```python
from build123d import *

# Parameters (mm, degrees)
SKETCH1_R                      = 88.9
BOSS_EXTRUDE1_DEPTH            = 3.175
SKETCH2_R                      = 12.065
BOSS_EXTRUDE2_DEPTH            = 3.175
SKETCH5_R                      = 10.4
CUT_EXTRUDE1_DEPTH             = 5.525
SKETCH6_R                      = 5
CUT_EXTRUDE2_DEPTH             = 4
CBORE_FOR_M2_SHCS1_D           = 2.2
CBORE_FOR_M2_SHCS1_DEPTH       = 6
CBORE_FOR_M2_SHCS1_CBORE_D     = 4.4
CBORE_FOR_M2_SHCS1_CBORE_DEPTH = 2
CBORE_FOR_M2_SHCS1_TIP         = 0.660946681
M4_CLEARANCE_HOLE1_D           = 4.5
CHAMFER1_SIZE                  = 5.08


with BuildPart() as part:
    # Sketch1 → Boss-Extrude1 (new, symmetric)
    with BuildSketch(Plane(origin=(0, 0, 0), x_dir=(1, 0, 0), z_dir=(0, 1, 0))):
        with Locations(Location((0, 0, 0), (0, 0, 270))):
            Circle(SKETCH1_R)
    extrude(amount=BOSS_EXTRUDE1_DEPTH, both=True)

    # Sketch2 → Boss-Extrude2 (add)
    with BuildSketch(Plane.XZ.offset(3.175)):
        with Locations(Location((0, 0, 0), (0, 0, 90))):
            Circle(SKETCH2_R)
    extrude(amount=BOSS_EXTRUDE2_DEPTH)

    # Sketch5 → Cut-Extrude1 (cut)
    with BuildSketch(Plane(origin=(0, 3.175, 0), x_dir=(1, 0, 0), z_dir=(0, 1, 0))):
        with Locations(Location((0, 0, 0), (0, 0, 270))):
            Circle(SKETCH5_R)
    extrude(amount=-CUT_EXTRUDE1_DEPTH, mode=Mode.SUBTRACT)

    # Sketch6 → Cut-Extrude2 (cut)
    with BuildSketch(Plane(origin=(0, -2.35, 0), x_dir=(1, 0, 0), z_dir=(0, 1, 0))):
        with Locations(Location((0, 0, 0), (0, 0, 270))):
            Circle(SKETCH6_R)
    extrude(amount=-CUT_EXTRUDE2_DEPTH, mode=Mode.SUBTRACT)

    # CBORE for M2 SHCS1
    with Locations(Plane(origin=(0, -2.35, 0), x_dir=(1, 0, 0), z_dir=(0, 1, 0))):
        with Locations((-5.65685425, 5.65685425), (0, 8), (5.65685425, 5.65685425), (8, 0), (5.65685425, -5.65685425), (0, -8), (-5.65685425, -5.65685425), (-8, 0)):
            CounterBoreHole(CBORE_FOR_M2_SHCS1_D / 2, CBORE_FOR_M2_SHCS1_CBORE_D / 2, CBORE_FOR_M2_SHCS1_CBORE_DEPTH, depth=CBORE_FOR_M2_SHCS1_DEPTH)
            with Locations((0, 0, -(CBORE_FOR_M2_SHCS1_DEPTH + CBORE_FOR_M2_SHCS1_TIP / 2))):  # 118° drill point
                Cone(0, CBORE_FOR_M2_SHCS1_D / 2, CBORE_FOR_M2_SHCS1_TIP, mode=Mode.SUBTRACT)

    # M4 Clearance Hole1 (through all)
    with Locations(Plane(origin=(0, 3.175, 0), x_dir=(1, 0, 0), z_dir=(0, 1, 0))):
        with Locations((19.05, -27.564242343), (-19.05, -27.564242343)):
            Hole(M4_CLEARANCE_HOLE1_D / 2)

    # Chamfer1
    chamfer1_edges = [part.edges().sort_by_distance(p)[0] for p in [
        (0, 3.175, -10.4),
    ]]
    chamfer(chamfer1_edges, length=CHAMFER1_SIZE)


solid = part.part
```
Design review of the part built by this model. Coordinates are the model's own, in mm. A direction names the side the tool comes from. Round coordinates to 2 decimals unless told otherwise and drop trailing zeros. Order: outer loops, then holes, each group sorted by start corner. A loop starts at its lowest first (then second) coordinate and runs counter-clockwise, first axis right, second up. Notation, with made-up numbers: (89, 18) - (137, 18) arc R34 ccw to (137, 51) - close; hole circle Ø10 at (31.5, 43.5). An arc over 180 degrees is marked (long way). One line per question, with ' | ' between items.
Item 1: Machinability: for faces 1 (the face through (-19, 3.175, -1)), 2 (the face through (-7, -4.35, 6)), which of the approach directions +Z, -Z, +X, -X, +Y, -Y give a long, thin tool a straight path to every point of the face, cutting with its end or side? Answer none if there is none.
Checks:
face 1: +Z, -Z, +X, -X, +Y | face 2: +Y
Item 2: Take a section at B-B, the plane y = 1.25. Write out the cut boundary in (x, z) (3 decimals), then the cut area to 3 significant figures.
Checks:
outline: circle Ø177.8 at (0, 0); hole circle Ø4.5 at (-19.05, 27.564); hole circle Ø27.11 at (0, 0); hole circle Ø4.5 at (19.05, 27.564) | area: 24,200 mm²
Item 3: Draft analysis for pull direction X (two halves, no side actions). For faces 3 (the face through (-17.26, -0.04, 28.93)), 4 (the face through (5.2, -6.35, -0.2)), state which applies: +X half, -X half, draft (parallel to the pull), parting line (faces both ways), or undercut.
Checks:
face 3: undercut | face 4: draft
Item 4: Take a section at C-C, the plane x = 59.5. Write out the cut boundary in (y, z) (3 decimals).
Checks:
outline: (-3.175, -66.053) - (3.175, -66.053) - (3.175, 66.053) - (-3.175, 66.053) - close
Item 5: Wall thickness on line 1 (X direction, y = -2.1, z = 0); line 2 (X direction, y = -1, z = 26); line 3 (Y direction, x = 20, z = -71.5) (3 decimals): over which ranges is each line inside the solid? List them lowest first. Write a range as [from, to].
Checks:
line 1: [-88.9, -10.4], [10.4, 88.9] | line 2: [-85.01, -20.67], [-17.43, 17.43], [20.67, 85.01] | line 3: [-3.175, 3.175]
Item 6: Take a section at A-A, the plane x = -19.05. Write out the cut boundary in (y, z) (3 decimals).
Checks:
outline: (-3.175, -86.835) - (3.175, -86.835) - (3.175, 25.314) - (-3.175, 25.314) - close; (-3.175, 29.814) - (3.175, 29.814) - (3.175, 86.835) - (-3.175, 86.835) - close
Item 7: Take a section at D-D, the plane z = 23. Write out the cut boundary in (x, y) (3 decimals).
Checks:
outline: (-85.873, -3.175) - (85.873, -3.175) - (85.873, 3.175) - (-85.873, 3.175) - close
Item 8: For P1, Ø3.5, axis at x = 1, z = -9, coming from the +Y side; P2, Ø8, axis at x = 39, z = 60.5, coming from the -Y side (3 decimals); P3, Ø5, axis at x = -6.5, z = 6, coming from the +Y side; P4, Ø1.8, axis at x = -5.66, z = -5.66, coming from the -Y side, all flat-tipped, find the tip position at first contact; note any pin that passes through.
Checks:
P1: y = -1.5 | P2: y = -3.175 | P3: y = -0.96 | P4: through
